Could you check a few things on this model? Use its own coordinates, in mm. A direction names the side the tool comes from. Give positions to 0.01 mm unless a question says otherwise; leave off trailing zeros. Loops run counter-clockwise (first coordinate to the right, second up) from the corner with the lowest first, then second, coordinate; pieces in that order, holes last. Notation, with made-up numbers: M 24,65 L 79,65 A19 ccw 79,82 Z; hole C 68.5,76 d10. An arc over 180 degrees is marked long. Use CSV: the item, a comma, the result in double quotes.
```python
from build123d import *

# Parameters (mm, degrees)
SKETCH1_W                      = 88.9
SKETCH1_H                      = 76.2
BASE_FLANGE1_DEPTH             = 6.35
EDGE_FLANGE1_START             = -44.45
EDGE_FLANGE1_DEPTH             = 88.9
EDGE_FLANGE1_2_DEPTH           = 88.9
F_7_0_201_DIAMETER_HOLE1_D     = 5.1054
F_7_0_201_DIAMETER_HOLE1_DEPTH = 6.35
FILLET1_R                      = 5.08


# Read off the part's stored shape, not the designer's step: Edge-Flange1
# Sheet-metal steps are written as plain solids
with BuildPart() as part:
    # Sketch1 → Base-Flange1 (new body)
    with BuildSketch(Plane(origin=(0, 0, 0), x_dir=(1, 0, 0), z_dir=(0, 1, 0))):
        Rectangle(SKETCH1_W, SKETCH1_H)
    extrude(amount=-BASE_FLANGE1_DEPTH)

    # Edge-Flange1 outline → Edge-Flange1 (cut)
    with BuildSketch(Plane.YZ.offset(EDGE_FLANGE1_START)):
        with BuildLine():
            Line((0, -38.1), (0, -35.625967843))
            ThreePointArc((0, -35.625967843), (-4.587857322, -32.419340017), (-6.35, -27.106548849))
            Line((-6.35, -27.106548849), (-6.35, -38.1))
            Line((-6.35, -38.1), (0, -38.1))
        make_face()
    extrude(amount=EDGE_FLANGE1_DEPTH, mode=Mode.SUBTRACT)

    # Edge-Flange1 2 outline → Edge-Flange1 2 (add)
    with BuildSketch(Plane.YZ.offset(EDGE_FLANGE1_START)):
        with BuildLine():
            ThreePointArc((0, -35.625967843), (3.190967678, -35.972683355), (6.297076347, -35.163625075))
            Line((6.297076347, -35.163625075), (200.831960117, 55.549481005))
            Line((200.831960117, 55.549481005), (198.148334155, 61.304535452))
            Line((198.148334155, 61.304535452), (3.613450385, -29.408570628))
            ThreePointArc((3.613450385, -29.408570628), (1.175258995, -29.248763121), (0, -27.106548849))
            Line((0, -27.106548849), (0, -35.625967843))
        make_face()
    extrude(amount=EDGE_FLANGE1_2_DEPTH)

    # #7 (0.201) Diameter Hole1
    with Locations(Plane(origin=(0, 0, 0), x_dir=(1, 0, 0), z_dir=(0, 1, 0))):
        with Locations((-34.9631, 19.05), (34.9631, 19.05), (34.9631, -31.75), (-34.9631, -31.75)):
            Hole(F_7_0_201_DIAMETER_HOLE1_D / 2, depth=F_7_0_201_DIAMETER_HOLE1_DEPTH)

    # Fillet1
    fillet1_edges = [part.edges().sort_by_distance(p)[0] for p in [
        (44.45, 199.490147136, 58.427008229),
        (-44.45, 199.490147136, 58.427008229),
        (44.45, -3.175, 38.1),
        (-44.45, -3.175, 38.1),
    ]]
    fillet(fillet1_edges, radius=FILLET1_R)


solid = part.part
```
1. If we mould it in two halves opening along X, with no side actions, what happens to faces 1 (the face through (36.99, -3.22, 33.3)), 2 (the face through (-1, 0, 5)), 3 (the face through (-36.141, -3.219, -16.785)), 4 (the face through (-44.45, 72, 1))? For each: +X half, -X half, draft (parallel to the pull), parting line (faces both ways), or undercut.
Outcome:
face 1,"undercut"
face 2,"draft"
face 3,"undercut"
face 4,"-X half"
2. I want a section at D-D, the plane y = 137.5. List the corners of the cut face in (x, z) for me.
Outcome:
outline,"M -44.45,26.02 L 44.45,26.02 L 44.45,33.02 L -44.45,33.02 Z"
3. Please list where these lines run through material, in increasing order: line 1 (X direction, y = -2, z = -19); line 2 (Y direction, x = -32, z = 21); line 3 (Y direction, x = 21, z = -26.5).
Outcome:
line 1,"-44.45 to -37.52, -32.41 to 32.41, 37.52 to 44.45"
line 2,"-6.35 to 0, 111.71 to 126.74"
line 3,"-6.35 to 0, 9.85 to 24.88"
4. I want a section at B-B, the plane x = -34.5. List the corners of the cut face in (y, z) for me.
Outcome:
outline,"M -6.35,-27.11 A8.89 ccw 6.3,-35.16 L 200.83,55.55 L 198.15,61.3 L 3.61,-29.41 A2.54 cw 0,-27.11 L 0,-21.56 L -6.35,-21.56 Z; M -6.35,-16.54 L 0,-16.54 L 0,29.24 L -6.35,29.24 Z; M -6.35,34.26 L 0,34.26 L 0,38.1 L -6.35,38.1 Z"
5. I want a section at C-C, the plane x = 14. List the corners of the cut face in (y, z) for me, then the cut area to 3 significant figures.
Outcome:
outline,"M -6.35,-27.11 A8.89 ccw 6.3,-35.16 L 200.83,55.55 L 198.15,61.3 L 3.61,-29.41 A2.54 cw 0,-27.11 L 0,38.1 L -6.35,38.1 Z"
area,"1,850 mm2"
6. I want a section at A-A, the plane z = -19.05. List the corners of the cut face in (x, y) for me.
Outcome:
outline,"M -44.45,-6.35 L -37.52,-6.35 L -37.52,0 L -44.45,0 Z; M -44.45,25.83 L 44.45,25.83 L 44.45,40.85 L -44.45,40.85 Z; M -32.41,-6.35 L 32.41,-6.35 L 32.41,0 L -32.41,0 Z; M 37.52,-6.35 L 44.45,-6.35 L 44.45,0 L 37.52,0 Z"
7. I'm going to push flat-ended pins straight in: pin 1 Ø6.5 at (x, z) = (34.96, -19.05) entering from +Y; pin 2 Ø3 at (x, y) = (4.5, -4) entering from +Z; pin 3 Ø3 at (x, z) = (-34.96, 31.75) entering from -Y; pin 4 Ø10 at (y, z) = (97.5, 25) entering from -X. Where does each tip first touch, or does it pass through?
Outcome:
pin 1,"y = 47.82"
pin 2,"z = 38.1"
pin 3,"y = 131.55"
pin 4,"through"
8. Which directions (+Z, -Z, +X, -X, +Y, -Y) give clear straight access to the entire face, cutting with the end or side of a thin tool? Please do faces 5 (the face through (-1, -3, 38.1)), 6 (the face through (-36.141, -3.219, 34.015)), 7 (the face through (-0.62, 102.24, 16.58)), 8 (the face through (43.001, -3.219, 36.572)).
Outcome:
face 5,"+Z, +X, -X, -Y"
face 6,"-Y"
face 7,"+Z, +X, -X"
face 8,"+Z, +X, -Y"
